from build123d import *

# Parameters (mm, degrees)
F0_R     = 15
F0_R_2   = 2.3
F1_DEPTH = 12
F0_R_3   = 48
F0_R_4   = 39.5
F2_DEPTH = 0.6
F3_SIZE  = 11.99999
F4_DEPTH = 6


# Not quite as in the source:
# - a fillet or chamfer is up to 0.001 mm smaller than in the source, because OpenCascade refuses the exact size


with BuildPart() as f1:
    # F0 (on Top) → F1 (new body)
    with BuildSketch(Plane.XY):
        Circle(F0_R)
        Circle(F0_R_2, mode=Mode.SUBTRACT)
    extrude(amount=F1_DEPTH)

    # F0 (on Top) → F2 (join)
    with BuildSketch(Plane.XY):
        Circle(F0_R_3)
        Circle(F0_R_4, mode=Mode.SUBTRACT)
        Circle(F0_R_4)
        Circle(F0_R, mode=Mode.SUBTRACT)
        Circle(F0_R)
        Circle(F0_R_2, mode=Mode.SUBTRACT)
    extrude(amount=-F2_DEPTH)

    # F3 (size 12 in the source; OpenCascade refuses exactly that, so slightly less here)
    f3_edges = [f1.edges().sort_by_distance(p)[0] for p in [
        (-15, 0, 12),
    ]]
    chamfer(f3_edges, length=F3_SIZE)

    # F0 (on Top) → F4 (join)
    with BuildSketch(Plane.XY):
        Circle(F0_R_3)
        Circle(F0_R_4, mode=Mode.SUBTRACT)
    extrude(amount=F4_DEPTH)


solid = f1.part
Work out the finished part from the listing and answer in its coordinate system (mm). A direction names the side the tool comes from. Give positions to 0.01 mm unless a question says otherwise; leave off trailing zeros. Loops run counter-clockwise (first coordinate to the right, second up) from the corner with the lowest first, then second, coordinate; pieces in that order, holes last. Notation, with made-up numbers: (36, -13.75) -> (90, -13.75) arc R21 cw to (90, 3.25) -> close; hole circle Ø11 at (87.25, -16.75). An arc over 180 degrees is marked (long way). Use a Markdown table: item, result. Add a question column.
1. Find the intervals of material crossed by probe 1 along X at (y, z) = (-3.5, 3.25); probe 2 along Y at (x, z) = (0, 4.5); probe 3 along Y at (x, z) = (0, 4), in increasing order.
2. Section C-C on z = 2.5 is taken. Determine the outline of the cut face in (x, y).
3. Flat-ended cylindrical pins translate along their axes: pin 1 Ø3 at (x, y) = (0, 0) entering from -Z; pin 2 Ø6 at (y, z) = (23, 4) entering from -X; pin 3 Ø2 at (x, y) = (-16, 27.5) entering from +Z; pin 4 Ø1.5 at (x, z) = (37, 3) entering from -Y. Find the tip coordinate at first contact, or state that the pin passes through.
4. Section D-D on x = 26 is taken. Determine the outline of the cut face in (y, z), and give its area (3 significant figures).
5. Determine the mould class of faces 3 (the flat face through (2, -2, 12)), 4 (the cylindrical face through (-1.825, -1.4, 5.612)) for opening direction X: released by +X, released by -X, zero draft, split by the parting line, or undercut.
6. For faces 1 (the flat face through (10, 1, -0.6)), 2 (the cylindrical face through (-29.11, 26.7, 2.96)), determine the directions among +Z, -Z, +X, -X, +Y, -Y from which every point of the face is accessible in a straight line to the end or side of a thin tool.
Results below:
| question | item | result |
|---|---|---|
| 1 | probe 1 | x = -47.87 to -39.34, -11.22 to 11.22, 39.34 to 47.87 |
| 1 | probe 2 | y = -48 to -39.5, -10.5 to -2.3, 2.3 to 10.5, 39.5 to 48 |
| 1 | probe 3 | y = -48 to -39.5, -11 to -2.3, 2.3 to 11, 39.5 to 48 |
| 2 | outline | circle Ø96 at (0, 0); circle Ø25 at (0, 0); hole circle Ø79 at (0, 0); hole circle Ø4.6 at (0, 0) |
| 3 | pin 1 | passes through |
| 3 | pin 2 | stops at x = -43.63 |
| 3 | pin 3 | stops at z = 0 |
| 3 | pin 4 | stops at y = -31.46 |
| 4 | outline | (-40.35, -0.6) -> (40.35, -0.6) -> (40.35, 6) -> (29.74, 6) -> (29.74, 0) -> (-29.74, 0) -> (-29.74, 6) -> (-40.35, 6) -> close |
| 4 | area | 176 mm^2 |
| 5 | face 3 | zero draft |
| 5 | face 4 | undercut |
| 6 | face 1 | -Z, +X, -X, +Y, -Y |
| 6 | face 2 | +Z |
